Work out the finished part from the listing and answer in its coordinate system (mm). A direction names the side the tool comes from. Give positions to 0.01 mm unless a question says otherwise; leave off trailing zeros. Loops run counter-clockwise (first coordinate to the right, second up) from the corner with the lowest first, then second, coordinate; pieces in that order, holes last. Notation, with made-up numbers: M 62.5,53.5 L 70.5,53.5 A15 ccw 70.5,62.5 Z; hole C -14,1.5 d3. An arc over 180 degrees is marked long. Answer as a JSON object with one key per item and string values. Group by question number.
```python
from build123d import *

# Parameters (mm, degrees)
SKETCH1_W                      = 405
SKETCH1_H                      = 29.5
BOSS_EXTRUDE1_DEPTH            = 2.54
EDGE_FLANGE1_STRIP_W           = 15.24
EDGE_FLANGE1_STRIP_H           = 2.54
EDGE_FLANGE1_STRIP_CUT_DEPTH   = 405
EDGE_FLANGE1_STRIP_2_W         = 15.24
EDGE_FLANGE1_STRIP_2_H         = 2.54
EDGE_FLANGE1_STRIP_CUT_2_DEPTH = 405
EDGE_FLANGE1_DEPTH             = 405
EDGE_FLANGE1_BEND_DEPTH        = 405
SKETCH17_R                     = 1.85
CUT_EXTRUDE1_DEPTH             = 206.186500531
CUT_EXTRUDE2_DEPTH             = 204.589814333
FILLET1_R                      = 1
FILLET2_R                      = 5


# Sheet-metal steps are written as plain solids
with BuildPart() as part:
    # Sketch1 → Boss-Extrude1 (new body)
    with BuildSketch(Plane(origin=(0, 0, 0), x_dir=(1, 0, 0), z_dir=(0, 1, 0))):
        Rectangle(SKETCH1_W, SKETCH1_H)
    extrude(amount=BOSS_EXTRUDE1_DEPTH)

    # Edge-Flange1 strip (across the edge) → Edge-Flange1 strip cut (cut)
    with BuildSketch(Plane(origin=(202.5, 2.54, -14.75), x_dir=(0, 0, 1), z_dir=(-1, 0, 0))):
        with Locations((-2.54, -1.27)):
            Rectangle(EDGE_FLANGE1_STRIP_W, EDGE_FLANGE1_STRIP_H)
    extrude(amount=EDGE_FLANGE1_STRIP_CUT_DEPTH, mode=Mode.SUBTRACT)

    # Edge-Flange1 strip 2 (across the edge) → Edge-Flange1 strip cut 2 (cut)
    with BuildSketch(Plane(origin=(-202.5, 2.54, 14.75), x_dir=(0, 0, -1), z_dir=(1, 0, 0))):
        with Locations((-2.54, -1.27)):
            Rectangle(EDGE_FLANGE1_STRIP_2_W, EDGE_FLANGE1_STRIP_2_H)
    extrude(amount=EDGE_FLANGE1_STRIP_CUT_2_DEPTH, mode=Mode.SUBTRACT)

    # Edge-Flange1 section (across the edge) → Edge-Flange1 (add)
    with BuildSketch(Plane(origin=(202.5, 2.54, -14.75), x_dir=(0, 0, 1), z_dir=(-1, 0, 0))):
        with BuildLine():
            Line((0, 2.54), (0, 12.46))
            Line((0, 12.46), (2.54, 12.46))
            Line((2.54, 12.46), (2.54, 2.54))
            ThreePointArc((2.54, 2.54), (3.283948776, 0.743948776), (5.08, 0))
            Line((5.08, 0), (5.08, -2.54))
            ThreePointArc((5.08, -2.54), (1.487897552, -1.052102448), (0, 2.54))
        make_face()
    extrude(amount=EDGE_FLANGE1_DEPTH)

    # Edge-Flange1 section 2 (across the edge) → Edge-Flange1 bend (add)
    with BuildSketch(Plane(origin=(-202.5, 2.54, 14.75), x_dir=(0, 0, -1), z_dir=(1, 0, 0))):
        with BuildLine():
            Line((0, 2.54), (0, 12.46))
            Line((0, 12.46), (2.54, 12.46))
            Line((2.54, 12.46), (2.54, 2.54))
            ThreePointArc((2.54, 2.54), (3.283948776, 0.743948776), (5.08, 0))
            Line((5.08, 0), (5.08, -2.54))
            ThreePointArc((5.08, -2.54), (1.487897552, -1.052102448), (0, 2.54))
        make_face()
    extrude(amount=EDGE_FLANGE1_BEND_DEPTH)

    # Sketch17 → Cut-Extrude1 (cut, through all)
    with BuildSketch(Plane.XY.offset(14.75)):
        with Locations((-197.33398, 10)):
            Circle(SKETCH17_R)
        with Locations((-98.66699, 10)):
            Circle(SKETCH17_R)
        with Locations((0, 10)):
            Circle(SKETCH17_R)
        with Locations((98.66699, 10)):
            Circle(SKETCH17_R)
        with Locations((197.33398, 10)):
            Circle(SKETCH17_R)
    extrude(amount=-CUT_EXTRUDE1_DEPTH, mode=Mode.SUBTRACT)

    # Sketch18 → Cut-Extrude2 (cut, through all)
    with BuildSketch(Plane.XZ):
        Polygon((-202.5, -4.67), (-132.5, -8), (-132.5, 8), (-202.5, 4.67), align=None)
    extrude(amount=-CUT_EXTRUDE2_DEPTH, mode=Mode.SUBTRACT)

    # Fillet1
    fillet1_edges = [part.edges().sort_by_distance(p)[0] for p in [
        (-202.5, 1.27, -4.67),
        (-202.5, 1.27, 4.67),
        (-132.5, 1.27, 8),
        (-132.5, 1.27, -8),
    ]]
    fillet(fillet1_edges, radius=FILLET1_R)

    # Fillet2
    fillet2_edges = [part.edges().sort_by_distance(p)[0] for p in [
        (202.5, 15, -13.48),
        (-202.5, 15, -13.48),
        (-202.5, 15, 13.48),
        (202.5, 15, 13.48),
    ]]
    fillet(fillet2_edges, radius=FILLET2_R)


solid = part.part
```
Item 1: A cutting plane is placed at A-A (x = -57). Determine the outline of the cut face in (y, z), and give its area (3 significant figures).
Item 2: Given pin 1 Ø4 at (x, z) = (160, 3.5) entering from +Y; pin 2 Ø0.8 at (y, z) = (1.5, 1) entering from -X; pin 3 Ø4 at (x, y) = (-18.5, 2) entering from -Z, each flat-ended and moving along its own axis, determine where each tip first touches the part or whether it passes through.
Item 3: A tool of negligible diameter and unlimited length cuts with its end or side. For faces 4 (the flat face through (-3, 10, 12.21)), 5 (the flat face through (202.5, 2, 0)), from which of +Z, -Z, +X, -X, +Y, -Y can it reach the whole face along a straight path? Write none if from no direction.
Item 4: For a pull along Z with two mould halves and no side action, classify faces 1 (the flat face through (3, 10, -14.75)), 2 (the flat face through (42, 2.54, 0)), 3 (the flat face through (42, 0, 0)) as pulls with the +Z half, pulls with the -Z half, needs draft (parallel to the pull), parting line crosses it, or undercut.
Item 5: A cutting plane is placed at B-B (x = -172.5). Determine the outline of the cut face in (y, z).
Item 6: Find the intervals of material crossed by probe 1 along Z at (x, y) = (179, 12.5); probe 2 along Y at (x, z) = (142.5, -7), in increasing order. Write a range as [from, to].
The answers:
{
 "1": {"outline": "M 0,-9.67 A5.08 ccw 5.08,-14.75 L 15,-14.75 L 15,-12.21 L 5.08,-12.21 A2.54 cw 2.54,-9.67 L 2.54,9.67 A2.54 cw 5.08,12.21 L 15,12.21 L 15,14.75 L 5.08,14.75 A5.08 ccw 0,9.67 Z", "area": "130 mm^2"},
 "2": {"pin 1": "stops at y = 2.54", "pin 2": "stops at x = -132.5", "pin 3": "stops at z = -14.63"},
 "3": {"face 4": "+X, -X, +Y", "face 5": "+Z, -Z, +X, +Y, -Y"},
 "4": {"face 1": "pulls with the -Z half", "face 2": "undercut", "face 3": "needs draft"},
 "5": {"outline": "M 0,-9.67 A5.08 ccw 5.08,-14.75 L 15,-14.75 L 15,-12.21 L 5.08,-12.21 A2.54 cw 2.54,-9.67 L 2.54,-6.1 L 0,-6.1 Z; M 0,6.1 L 2.54,6.1 L 2.54,9.67 A2.54 cw 5.08,12.21 L 15,12.21 L 15,14.75 L 5.08,14.75 A5.08 ccw 0,9.67 Z"},
 "6": {"probe 1": "z = [-14.75, -12.21], [12.21, 14.75]", "probe 2": "y = [0, 2.54]"}
}
